The model under review builds one solid part; all positions refer to its coordinate system, in mm. A direction names the side the tool comes from. Give positions to 0.01 mm unless a question says otherwise; leave off trailing zeros. Order: outer loops, then holes, each group sorted by start corner. A loop starts at its lowest first (then second) coordinate and runs counter-clockwise, first axis right, second up. Notation, with made-up numbers: (14, 73) -> (45, 73) arc R32 cw to (45, 112) -> close; hole circle Ø10 at (-26, 11.25). An arc over 180 degrees is marked (long way). Answer as a JSON object with one key per item and string values. Group by question number.
from build123d import *

# Parameters (mm, degrees)
SKETCH001_R  = 5.5
POCKET_DEPTH = 7.001
CHAMFER_SIZE = 0.4


with BuildPart() as part:
    # Sketch → Revolution (revolve)
    with BuildSketch(Plane.XY):
        Polygon((30, 0), (30, 7), (9, 7), (9, 5), (12.8, 5), (12.8, 0), align=None)
    revolve(axis=Axis((0, 0, 0), (0, 1, 0)))

    # Sketch001 (on Face6 of Revolution) → Pocket (cut, through all)
    with BuildSketch(Plane.XZ):
        with Locations((0.124373, 21.635731)):
            Circle(SKETCH001_R)
        with Locations((15.386717, 15.210827)):
            Circle(SKETCH001_R)
        with Locations((21.635731, -0.124373)):
            Circle(SKETCH001_R)
        with Locations((15.210827, -15.386717)):
            Circle(SKETCH001_R)
        with Locations((-0.124373, -21.635731)):
            Circle(SKETCH001_R)
        with Locations((-15.386717, -15.210827)):
            Circle(SKETCH001_R)
        with Locations((-21.635731, 0.124373)):
            Circle(SKETCH001_R)
        with Locations((-15.210827, 15.386717)):
            Circle(SKETCH001_R)
    extrude(amount=-POCKET_DEPTH, mode=Mode.SUBTRACT)

    # Chamfer
    chamfer_edges = [part.edges().sort_by_distance(p)[0] for p in [
        (-12.8, 0, 0),
    ]]
    chamfer(chamfer_edges, length=CHAMFER_SIZE)


solid = part.part
1. Take a section at B-B on x = 24. Give the boundary of the cut face in (y, z), plus the area to 3 significant figures.
2. Draft analysis for pull direction X (two halves, no side actions). For faces 1 (the flat face through (-13, 0, 6)), 2 (the cylindrical face through (-29.97, 3.55, -1.32)), 3 (the cylindrical face through (18.34, 3.45, 19.85)), state which applies: pulls with the +X half, pulls with the -X half, needs draft (parallel to the pull), parting line crosses it, or undercut.
3. For pin 1 (9 mm diameter, centred on x = 0.12, z = 21.64, fed in from +Y); pin 2 (1.5 mm diameter, centred on y = 5, z = 18, fed in from -X); pin 3 (20.5 mm diameter, centred on x = 0, z = 0, fed in from -Y), all flat-tipped, find the tip position at first contact; note any pin that passes through.
4. Take a section at A-A on x = 14. Give the boundary of the cut face in (y, z), plus the area to 3 significant figures.
5. For probe 1 along X at (y, z) = (5.7, 0); probe 2 along X at (y, z) = (6, 15), list the stretches that pass through material, from the lowest coordinate up. Write a range as [from, to].
6. Take a section at D-D on x = 0. Give the boundary of the cut face in (y, z).
7. Take a section at C-C on y = 6. State how many separate pieces and enclosed holes the cut face has, plus the area to 3 significant figures.
8. Machinability: for faces 4 (the cylindrical face through (-0.59, 3.45, 27.09)), 5 (the cylindrical face through (-10.158, 2.668, 7.789)), which of the approach directions +Z, -Z, +X, -X, +Y, -Y give a long, thin tool a straight path to every point of the face, cutting with its end or side? Answer none if there is none.
Checks:
{
 "1": {"outline": "(0, -18) -> (7, -18) -> (7, -5.09) -> (0, -5.09) -> close; (0, 4.84) -> (7, 4.84) -> (7, 18) -> (0, 18) -> close", "area": "182 mm2"},
 "2": {"face 1": "needs draft", "face 2": "parting line crosses it", "face 3": "undercut"},
 "3": {"pin 1": "passes through", "pin 2": "stops at x = -24.54", "pin 3": "stops at y = 5"},
 "4": {"outline": "(0, -26.53) -> (7, -26.53) -> (7, -20.75) -> (0, -20.75) -> close; (0, -10.02) -> (7, -10.02) -> (7, 9.89) -> (0, 9.89) -> close; (0, 20.53) -> (7, 20.53) -> (7, 26.53) -> (0, 26.53) -> close", "area": "222 mm2"},
 "5": {"probe 1": "x = [-30, -27.13], [-16.14, -9], [9, 16.14], [27.13, 30]", "probe 2": "x = [-25.98, -20.7], [-9.72, 9.89], [20.88, 25.98]"},
 "6": {"outline": "(0, -30) -> (7, -30) -> (7, -27.13) -> (0, -27.13) -> close; (0, -16.14) -> (7, -16.14) -> (7, -9) -> (5, -9) -> (5, -12.8) -> (0.4, -12.8) -> (0, -13.2) -> close; (0, 13.2) -> (0.4, 12.8) -> (5, 12.8) -> (5, 9) -> (7, 9) -> (7, 16.14) -> (0, 16.14) -> close; (0, 27.13) -> (7, 27.13) -> (7, 30) -> (0, 30) -> close"},
 "7": {"separate pieces": "1", "enclosed holes": "9", "area": "1,810 mm2"},
 "8": {"face 4": "+Y, -Y", "face 5": "-Y"}
}
